Verification items for the finished model (mm, model axes). A direction names the side the tool comes from. Round coordinates to 2 decimals unless told otherwise and drop trailing zeros. Loops run counter-clockwise (first coordinate to the right, second up) from the corner with the lowest first, then second, coordinate; pieces in that order, holes last. Notation, with made-up numbers: (56.25, -3) -> (86.25, -3) arc R10 cw to (86.25, 1) -> close; hole circle Ø3 at (5, 74.25). An arc over 180 degrees is marked (long way). Write item = value, one per line.
```python
from build123d import *

# Parameters (mm, degrees)
F1_DEPTH = 4


with BuildPart() as f1:
    # F0 (on Right) → F1 (new body)
    with BuildSketch(Plane.YZ):
        Polygon((17.2320508076, -23.8467875173), (29.2679491924, -3), (23.2679491924, -3), (23.2679491924, 3), (29.2679491924, 3), (17.2320508076, 23.8467875173), (14.2320508076, 18.6506350946), (9.0358983849, 21.6506350946), (12.0358983849, 26.8467875173), (-12.0358983849, 26.8467875173), (-9.0358983849, 21.6506350946), (-14.2320508076, 18.6506350946), (-17.2320508076, 23.8467875173), (-29.2679491924, 3), (-23.2679491924, 3), (-23.2679491924, -3), (-29.2679491924, -3), (-17.2320508076, -23.8467875173), (-14.2320508076, -18.6506350946), (-9.0358983849, -21.6506350946), (-12.0358983849, -26.8467875173), (12.0358983849, -26.8467875173), (9.0358983849, -21.6506350946), (14.2320508076, -18.6506350946), align=None)
        with BuildLine():
            ThreePointArc((17.2409396496, 3), (17.4351146235, 1.5055823014), (17.5, 0))
            ThreePointArc((17.5, 0), (17.4351146235, -1.5055823014), (17.2409396496, -3))
            ThreePointArc((17.2409396496, -3), (15.1554445662, -8.75), (11.2185460361, -13.4310917216))
            ThreePointArc((11.2185460361, -13.4310917216), (8.75, -15.1554445662), (6.0223936134, -16.4310917216))
            ThreePointArc((6.0223936134, -16.4310917216), (0, -17.5), (-6.0223936134, -16.4310917216))
            ThreePointArc((-6.0223936134, -16.4310917216), (-8.75, -15.1554445662), (-11.2185460361, -13.4310917216))
            ThreePointArc((-11.2185460361, -13.4310917216), (-15.1554445662, -8.75), (-17.2409396496, -3))
            ThreePointArc((-17.2409396496, -3), (-17.5, 0), (-17.2409396496, 3))
            ThreePointArc((-17.2409396496, 3), (-15.1554445662, 8.75), (-11.2185460361, 13.4310917216))
            ThreePointArc((-11.2185460361, 13.4310917216), (-8.75, 15.1554445662), (-6.0223936134, 16.4310917216))
            ThreePointArc((-6.0223936134, 16.4310917216), (0, 17.5), (6.0223936134, 16.4310917216))
            ThreePointArc((6.0223936134, 16.4310917216), (8.75, 15.1554445662), (11.2185460361, 13.4310917216))
            ThreePointArc((11.2185460361, 13.4310917216), (15.1554445662, 8.75), (17.2409396496, 3))
        make_face(mode=Mode.SUBTRACT)
        with BuildLine():
            ThreePointArc((17.2409396496, -3), (17.4351146235, -1.5055823014), (17.5, 0))
            ThreePointArc((17.5, 0), (17.4351146235, 1.5055823014), (17.2409396496, 3))
            Line((17.2409396496, 3), (5.1961524227, 3))
            Line((5.1961524227, 3), (3.4641016151, 0))
            Line((3.4641016151, 0), (5.1961524227, -3))
            Line((5.1961524227, -3), (17.2409396496, -3))
        make_face()
        with BuildLine():
            Line((5.1961524227, 3), (11.2185460361, 13.4310917216))
            ThreePointArc((11.2185460361, 13.4310917216), (8.75, 15.1554445662), (6.0223936134, 16.4310917216))
            Line((6.0223936134, 16.4310917216), (0, 6))
            Line((0, 6), (1.7320508076, 3))
            Line((1.7320508076, 3), (5.1961524227, 3))
        make_face()
        Polygon((3.4641016151, 0), (5.1961524227, 3), (1.7320508076, 3), align=None)
        with BuildLine():
            ThreePointArc((6.0223936134, -16.4310917216), (8.75, -15.1554445662), (11.2185460361, -13.4310917216))
            Line((11.2185460361, -13.4310917216), (5.1961524227, -3))
            Line((5.1961524227, -3), (1.7320508076, -3))
            Line((1.7320508076, -3), (0, -6))
            Line((0, -6), (6.0223936134, -16.4310917216))
        make_face()
        Polygon((1.7320508076, -3), (5.1961524227, -3), (3.4641016151, 0), align=None)
        Polygon((-1.7320508076, 3), (1.7320508076, 3), (0, 6), align=None)
        Polygon((3.4641016151, 0), (1.7320508076, 3), (-1.7320508076, 3), (-3.4641016151, 0), (-1.7320508076, -3), (1.7320508076, -3), align=None)
        Polygon((0, -6), (1.7320508076, -3), (-1.7320508076, -3), align=None)
        with BuildLine():
            Line((0, 6), (-6.0223936134, 16.4310917216))
            ThreePointArc((-6.0223936134, 16.4310917216), (-8.75, 15.1554445662), (-11.2185460361, 13.4310917216))
            Line((-11.2185460361, 13.4310917216), (-5.1961524227, 3))
            Line((-5.1961524227, 3), (-1.7320508076, 3))
            Line((-1.7320508076, 3), (0, 6))
        make_face()
        Polygon((-3.4641016151, 0), (-1.7320508076, 3), (-5.1961524227, 3), align=None)
        with BuildLine():
            ThreePointArc((-11.2185460361, -13.4310917216), (-8.75, -15.1554445662), (-6.0223936134, -16.4310917216))
            Line((-6.0223936134, -16.4310917216), (0, -6))
            Line((0, -6), (-1.7320508076, -3))
            Line((-1.7320508076, -3), (-5.1961524227, -3))
            Line((-5.1961524227, -3), (-11.2185460361, -13.4310917216))
        make_face()
        Polygon((-5.1961524227, -3), (-1.7320508076, -3), (-3.4641016151, 0), align=None)
        with BuildLine():
            Line((-3.4641016151, 0), (-5.1961524227, 3))
            Line((-5.1961524227, 3), (-17.2409396496, 3))
            ThreePointArc((-17.2409396496, 3), (-17.5, 0), (-17.2409396496, -3))
            Line((-17.2409396496, -3), (-5.1961524227, -3))
            Line((-5.1961524227, -3), (-3.4641016151, 0))
        make_face()
    extrude(amount=F1_DEPTH)


solid = f1.part
```
(1) Material ranges on probe 1 along Y at (x, z) = (1, 4.5); probe 2 along Y at (x, z) = (0.35, 3.5); probe 3 along Y at (x, z) = (0.45, 8.5), recorded low to high. Write a range as from..to.
Filled sheet:
probe_1 = -28.4..-16.91, -6.06..6.06, 16.91..28.4
probe_2 = -28.98..-17.15, -5.48..5.48, 17.15..28.98
probe_3 = -26.09..-15.3, -8.37..-1.44, 1.44..8.37, 15.3..26.09
(2) Sectioned sample at C-C, the plane x = 1.7. Count the separate pieces of the cut face and the enclosed holes in it, and give its area (3 significant figures).
Filled sheet:
separate_pieces = 1
enclosed_holes = 6
area = 1,820 mm2
(3) Go/stop test with flat-tipped pins: pin 1 Ø2 at (y, z) = (-16, -6.5) entering from -X; pin 2 Ø1.2 at (x, y) = (3, -26) entering from +Z; pin 3 Ø1.2 at (x, y) = (1.5, -27) entering from -Z; pin 4 Ø1.2 at (x, y) = (2, 27.5) entering from +Z. Record where each tip stops, or that it passes through.
Filled sheet:
pin_1 = 0
pin_2 = 9.7
pin_3 = -7.97
pin_4 = 7.1
(4) Sectioned sample at B-B, the plane z = -7. Record the cut outline in (x, y).
Filled sheet:
outline = (0, -26.96) -> (4, -26.96) -> (4, -16.04) -> (0, -16.04) -> close; (0, -7.51) -> (4, -7.51) -> (4, -0.58) -> (0, -0.58) -> close; (0, 0.58) -> (4, 0.58) -> (4, 7.51) -> (0, 7.51) -> close; (0, 16.04) -> (4, 16.04) -> (4, 26.96) -> (0, 26.96) -> close
(5) Draft check along Z on faces 5 (the face through (1.972, -23.166, 13.569)), 6 (the face through (0, 0, 0)), 7 (the face through (1.972, -15.198, 8.675)). Enter one of: released by +Z, released by -Z, zero draft, split by the parting line, or undercut.
Filled sheet:
face_5 = released by +Z
face_6 = zero draft
face_7 = undercut
(6) Sectioned sample at A-A, the plane z = 20. Record the cut outline in (x, y).
Filled sheet:
outline = (0, -19.45) -> (4, -19.45) -> (4, -15.01) -> (0, -15.01) -> close; (0, -11.89) -> (4, -11.89) -> (4, 11.89) -> (0, 11.89) -> close; (0, 15.01) -> (4, 15.01) -> (4, 19.45) -> (0, 19.45) -> close
(7) Sectioned sample at D-D, the plane z = 2. Record the cut outline in (x, y).
Filled sheet:
outline = (0, -23.27) -> (4, -23.27) -> (4, 23.27) -> (0, 23.27) -> close
(8) Set-up check for faces 1 (the face through (1.972, 23.334, 13.277)), 2 (the face through (1.97, 8.25, -8.29)), 3 (the face through (2, -23.268, 0)), 4 (the face through (2, 26, -3)): record each of +Z, -Z, +X, -X, +Y, -Y from which the full face is reachable in a straight line by a thin tool's end or side.
Filled sheet:
face_1 = +Z, +X, -X, +Y
face_2 = +X, -X
face_3 = +X, -X, -Y
face_4 = +X, -X, +Y
